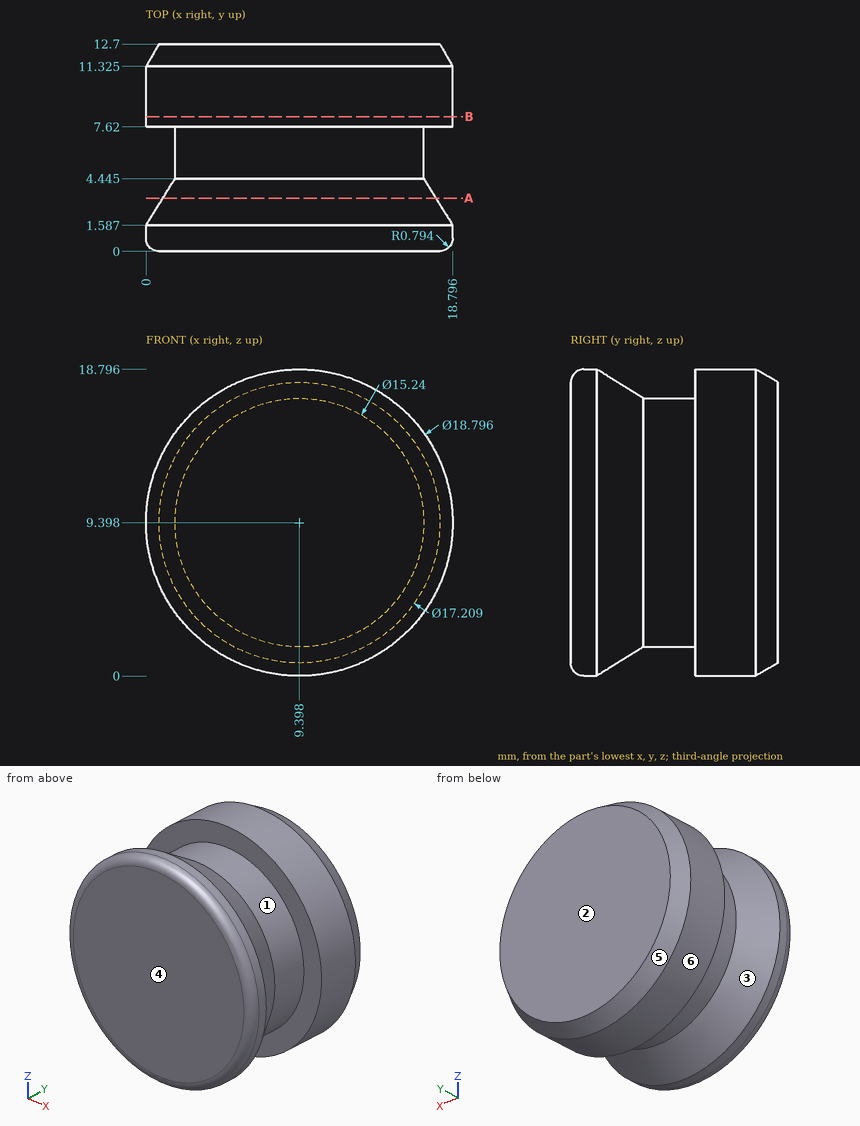
Geometry: see drawing. Coordinates: mm, zero at the bounding-box minimum. A direction names the side the tool comes from. Coordinates: 2 decimals unless noted, no trailing zeros. Loops run counter-clockwise (first coordinate to the right, second up) from the corner with the lowest first, then second, coordinate; pieces in that order, holes last.
(1) Pull-direction query (Y, two-part tool) for the marked faces 3, 4, 5 and 6; classes: released by +Y, released by -Y, zero draft, split by the parting line, or undercut.
(2) Section A-A on y = 3.25. Return the cut outline in (x, z) (1 decimal), then the cut area to 3 significant figures.
(3) First-contact query: pin 1 Ø5 at (y, z) = (8, 16.5) entering from +X; pin 2 Ø3 at (y, z) = (8.5, 16) entering from -X (1 decimal); pin 3 Ø6 at (x, z) = (5.5, 16.5) entering from -Y; pin 4 Ø2 at (x, y) = (6, 2.5) entering from +Z. Flat tips, straight axial feed; report the tip coordinate or a pass-through.
(4) Set-up query: the marked faces 1 and 2. Return all of +Z, -Z, +X, -X, +Y, -Y with unobstructed straight access to the full face (end or side cutting, diameter ignored); none if empty.
(5) Material intervals for probe 1 along Y at (x, z) = (3.5, 2.5) (1 decimal); probe 2 along Y at (x, z) = (17.5, 7.5) (1 decimal); probe 3 along X at (y, z) = (6, 9.25), sorted ascending.
(6) Section B-B on y = 8.25. Return the cut outline in (x, z) (1 decimal).
Data:
1. face 3: undercut
1. face 4: released by -Y
1. face 5: released by +Y
1. face 6: zero draft
2. outline: circle Ø16.7 at (9.4, 9.4)
2. area: 220 mm2
3. pin 1: stops at x = 17.59
3. pin 2: stops at x = 1.5
3. pin 3: stops at y = 0
3. pin 4: stops at z = 18.31
4. face 1: none
4. face 2: +Z, -Z, +X, -X, +Y
5. probe 1: y = 0.2 to 2.1, 7.6 to 11.9
5. probe 2: y = 0 to 3.3, 7.6 to 12.7
5. probe 3: x = 1.78 to 17.02
6. outline: circle Ø18.8 at (9.4, 9.4)
